Answer from the drawing. Dimensions are ordinates in mm from the lowest x, y and z of the part. A direction names the side the tool comes from. Give positions to 0.01 mm unless a question says otherwise; leave off trailing zeros. Order: outer loops, then holes, each group sorted by start corner. A loop starts at its lowest first (then second) coordinate and runs counter-clockwise, first axis right, second up.
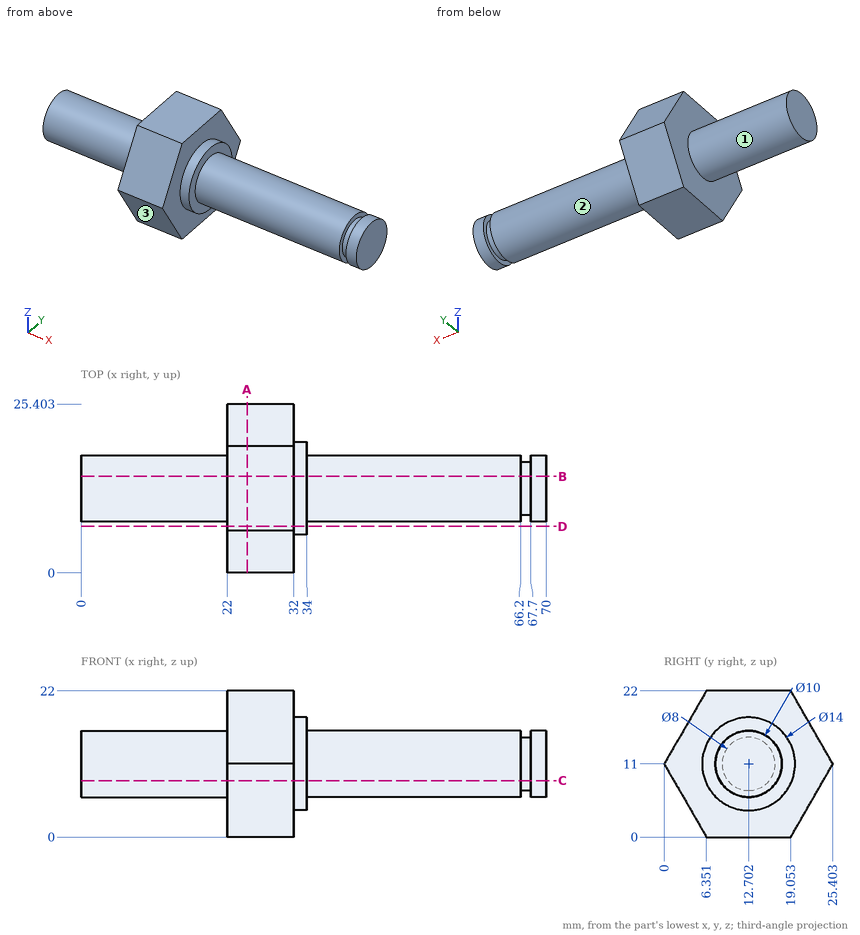
1) The part is cut by section A-A on x = 25. Determine the outline of the cut face in (y, z), and give its area (3 significant figures).
Final values:
outline: (0, 11) - (6.35, 0) - (19.05, 0) - (25.4, 11) - (19.05, 22) - (6.35, 22) - close
area: 419 mm2
2) A tool of negligible diameter and unlimited length cuts with its end or side. For the marked faces 1, 2 and 3, from which of +Z, -Z, +X, -X, +Y, -Y can it reach the whole face along a straight path? Write none if from no direction.
Final values:
face 1: -X
face 2: +X
face 3: -Z, +X, -X, -Y
3) Given pin 1 (10 mm diameter, centred on x = 37.5, z = 6, fed in from +Y) (1 decimal); pin 2 (1.5 mm diameter, centred on y = 15.5, z = 14.5, fed in from -X); pin 3 (8 mm diameter, centred on x = 13, y = 11, fed in from +Z); pin 4 (1 mm diameter, centred on y = 3, z = 14, fed in from -X), each flat-ended and moving along its own axis, determine where each tip first touches the part or whether it passes through.
Final values:
pin 1: stops at y = 19.6
pin 2: stops at x = 0
pin 3: stops at z = 16
pin 4: stops at x = 22
4) The part is cut by section C-C on z = 8.5. Determine the outline of the cut face in (x, y) (1 decimal).
Final values:
outline: (0, 8.4) - (22, 8.4) - (22, 1.4) - (32, 1.4) - (32, 6.2) - (34, 6.2) - (34, 8.4) - (66.2, 8.4) - (66.2, 9.6) - (67.7, 9.6) - (67.7, 8.4) - (70, 8.4) - (70, 17) - (67.7, 17) - (67.7, 15.8) - (66.2, 15.8) - (66.2, 17) - (34, 17) - (34, 19.2) - (32, 19.2) - (32, 24) - (22, 24) - (22, 17) - (0, 17) - close
5) The part is cut by section D-D on y = 7. Determine the outline of the cut face in (x, z).
Final values:
outline: (22, 0) - (32, 0) - (32, 6.94) - (34, 6.94) - (34, 15.06) - (32, 15.06) - (32, 22) - (22, 22) - close
6) Consider L1, parallel to X at y = 20.5, z = 14.5; L2, parallel to X at y = 13, z = 15.25; L3, parallel to X at y = 15.75, z = 16.25. Determine where each line is inside the solid, lowest interval first.
Final values:
L1: x = 22 to 32
L2: x = 0 to 66.2, 67.7 to 70
L3: x = 22 to 34
7) The part is cut by section B-B on y = 14.5. Determine the outline of the cut face in (x, z) (1 decimal).
Final values:
outline: (0, 6.3) - (22, 6.3) - (22, 0) - (32, 0) - (32, 4.2) - (34, 4.2) - (34, 6.3) - (66.2, 6.3) - (66.2, 7.4) - (67.7, 7.4) - (67.7, 6.3) - (70, 6.3) - (70, 15.7) - (67.7, 15.7) - (67.7, 14.6) - (66.2, 14.6) - (66.2, 15.7) - (34, 15.7) - (34, 17.8) - (32, 17.8) - (32, 22) - (22, 22) - (22, 15.7) - (0, 15.7) - close
